```python
from build123d import *

# Parameters (mm, degrees)
ESQUISSE1_R          = 3
ESQUISSE1_R_2        = 2.7
BOSS_EXTRU_1_DEPTH   = 1.25
ESQUISSE1_R_3        = 1.8
ESQUISSE1_R_4        = 1.5
BOSS_EXTRU_1_2_DEPTH = 1.25
ESQUISSE2_R          = 2.7
ESQUISSE2_R_2        = 1.8
BOSS_EXTRU_2_DEPTH   = 1.15


with BuildPart() as part:
    # Esquisse1 → Boss.-Extru.1 (new, symmetric)
    with BuildSketch(Plane(origin=(0, 0, 0), x_dir=(0, 0, -1), z_dir=(1, 0, 0))):
        Circle(ESQUISSE1_R)
        Circle(ESQUISSE1_R_2, mode=Mode.SUBTRACT)
    extrude(amount=BOSS_EXTRU_1_DEPTH, both=True)



with BuildPart() as body_2:
    # Esquisse1 → Boss.-Extru.1 2 (new, symmetric)
    with BuildSketch(Plane(origin=(0, 0, 0), x_dir=(0, 0, -1), z_dir=(1, 0, 0))):
        Circle(ESQUISSE1_R_3)
        Circle(ESQUISSE1_R_4, mode=Mode.SUBTRACT)
    extrude(amount=BOSS_EXTRU_1_2_DEPTH, both=True)


with BuildPart() as part_1:
    add(part.part)

    add(body_2.part)  # Boss.-Extru.2 merges body 2
    # Esquisse2 → Boss.-Extru.2 (add, symmetric)
    with BuildSketch(Plane(origin=(0, 0, 0), x_dir=(0, 0, -1), z_dir=(1, 0, 0))):
        Circle(ESQUISSE2_R)
        Circle(ESQUISSE2_R_2, mode=Mode.SUBTRACT)
    extrude(amount=BOSS_EXTRU_2_DEPTH, both=True)


solid = part_1.part
```
Could you check a few things on this model? Use its own coordinates, in mm. A direction names the side the tool comes from. Round coordinates to 2 decimals unless told otherwise and drop trailing zeros. Write each loop counter-clockwise with the first axis right and the second up, starting at its lowest first coordinate (ties: lowest second). Pieces come first, ordered by that corner, then holes.
(1) Suppose I cut it at A-A on z = 0. Write out the boundary of the cut face in (x, y).
Findings below:
outline: (-1.25, -3) - (1.25, -3) - (1.25, -2.7) - (1.15, -2.7) - (1.15, -1.8) - (1.25, -1.8) - (1.25, -1.5) - (-1.25, -1.5) - (-1.25, -1.8) - (-1.15, -1.8) - (-1.15, -2.7) - (-1.25, -2.7) - close; (-1.25, 1.5) - (1.25, 1.5) - (1.25, 1.8) - (1.15, 1.8) - (1.15, 2.7) - (1.25, 2.7) - (1.25, 3) - (-1.25, 3) - (-1.25, 2.7) - (-1.15, 2.7) - (-1.15, 1.8) - (-1.25, 1.8) - close
(2) For pin 1 (2.5 mm diameter, centred on y = -0.5, z = -1, fed in from -X); pin 2 (1.5 mm diameter, centred on x = 0, y = 1.5, fed in from -Z); pin 3 (1 mm diameter, centred on x = 0.5, y = 1, fed in from -Z), each with a flat end and sliding along its axis, tell me the tip position at first contact or that it passes through.
Findings below:
pin 1: stops at x = -1.25
pin 2: stops at z = -2.9
pin 3: stops at z = -2.96
(3) Thinking about a two-plate mould opening in Y: for faces 1 (the face through (1.15, -1, -2)), 2 (the face through (0, 0, 3)), which applies, +Y half, -Y half, draft (parallel to the pull), parting line (faces both ways), or undercut?
Findings below:
face 1: undercut
face 2: parting line
(4) Suppose I cut it at C-C on x = 0.35. Write out the boundary of the cut face in (y, z).
Findings below:
outline: circle Ø6 at (0, 0); hole circle Ø3 at (0, 0)
(5) Which directions (+Z, -Z, +X, -X, +Y, -Y) give clear straight access to the entire face, cutting with the end or side of a thin tool? Please do faces 3 (the face through (-1.15, -1, -2)), 4 (the face through (-0.02, 0.07, 1.5)).
Findings below:
face 3: -X
face 4: +X, -X
(6) If I drill on probe 1 along Y at (x, z) = (1.2, 0); probe 2 along Y at (x, z) = (-0.45, 0); probe 3 along X at (y, z) = (1.4, 2.2), over which ranges is the centre line in solid material (lowest first)?
Findings below:
probe 1: y = -3 to -2.7, -1.8 to -1.5, 1.5 to 1.8, 2.7 to 3
probe 2: y = -3 to -1.5, 1.5 to 3
probe 3: x = -1.15 to 1.15
(7) Suppose I cut it at D-D on z = -2.4. Write out the boundary of the cut face in (x, y), and give its area (3 significant figures).
Findings below:
outline: (-1.25, -1.8) - (1.25, -1.8) - (1.25, -1.24) - (1.15, -1.24) - (1.15, 1.24) - (1.25, 1.24) - (1.25, 1.8) - (-1.25, 1.8) - (-1.25, 1.24) - (-1.15, 1.24) - (-1.15, -1.24) - (-1.25, -1.24) - close
area: 8.51 mm2
